Here's how the part is built. I have some questions about the finished solid (model axes, mm). Face numbers are marked on the shaded views. A direction names the side the tool comes from. Round coordinates to 2 decimals unless told otherwise and drop trailing zeros. Loops run counter-clockwise (first coordinate to the right, second up) from the corner with the lowest first, then second, coordinate; pieces in that order, holes last. Notation, with made-up numbers: M 67,10 L 126,10 A26 cw 126,41 Z; hole C -22,-33.75 d10. An arc over 180 degrees is marked long. Answer as a JSON object with one key per item and string values.
from build123d import *

# Parameters (mm, degrees)
SKETCH1_R           = 3.25
BOSS_EXTRUDE1_DEPTH = 2.25
SKETCH2_R           = 3.25
BOSS_EXTRUDE2_DEPTH = 5
SKETCH3_R           = 3.25
CUT_EXTRUDE1_DEPTH  = 26.744736797
FILLET1_R           = 5
CHAMFER1_SIZE       = 1
CUT_EXTRUDE2_REACH  = 52.824
SKETCH4_R           = 1.35
CHAMFER2_SIZE       = 0.75
CHAMFER2_SIZE2      = 2.060608065
CHAMFER3_SIZE       = 1


with BuildPart() as part:
    # Sketch1 → Boss-Extrude1 (new body, symmetric)
    with BuildSketch(Plane(origin=(0, 0, 0), x_dir=(0, 0, -1), z_dir=(1, 0, 0))):
        with BuildLine():
            Line((-1.775856455, 11.411388509), (3.7711595, 19.333348288))
            ThreePointArc((3.7711595, 19.333348288), (14.912987345, 21.297953152), (16.877592209, 10.156125306))
            Line((16.877592209, 10.156125306), (6.553216354, -4.588611491))
            ThreePointArc((6.553216354, -4.588611491), (3.693988906, -7.096086665), (0, -8))
            Line((0, -8), (-12.5, -8))
            Line((-12.5, -8), (-12.5, -3))
            Line((-12.5, -3), (-32.5, -3))
            Line((-32.5, -3), (-32.5, 8))
            Line((-32.5, 8), (-25, 8))
            Line((-25, 8), (-8.329072809, 8))
            ThreePointArc((-8.329072809, 8), (-4.635083903, 8.903913335), (-1.775856455, 11.411388509))
        make_face()
        Circle(SKETCH1_R, mode=Mode.SUBTRACT)
        with Locations((10.324375854, 14.744736797)):
            Circle(SKETCH1_R, mode=Mode.SUBTRACT)
    extrude(amount=BOSS_EXTRUDE1_DEPTH, both=True)

    # Sketch2 → Boss-Extrude2 (add)
    with BuildSketch(Plane(origin=(2.25, 0, 0), x_dir=(0, 0, -1), z_dir=(1, 0, 0))):
        with BuildLine():
            Line((-32.5, 8), (0, 8))
            ThreePointArc((0, 8), (8, 0), (0, -8))
            Line((0, -8), (-12.5, -8))
            Line((-12.5, -8), (-12.5, -3))
            Line((-12.5, -3), (-32.5, -3))
            Line((-32.5, -3), (-32.5, 8))
        make_face()
        Circle(SKETCH2_R, mode=Mode.SUBTRACT)
    boss_extrude2 = extrude(amount=BOSS_EXTRUDE2_DEPTH)

    # Mirror1: Boss-Extrude2 across plane
    add(boss_extrude2.mirror(Plane(origin=(0, 0, 0), x_dir=(0, 0, 1), z_dir=(1, 0, 0))))

    # Sketch3 → Cut-Extrude1 (cut, through all)
    with BuildSketch(Plane.XZ.offset(3)):
        with Locations((0, 25)):
            Circle(SKETCH3_R)
    extrude(amount=-CUT_EXTRUDE1_DEPTH, mode=Mode.SUBTRACT)

    # Fillet1
    fillet1_edges = [part.edges().sort_by_distance(p)[0] for p in [
        (7.25, 2.5, 32.5),
        (-7.25, 2.5, 32.5),
    ]]
    fillet(fillet1_edges, radius=FILLET1_R)

    # Chamfer1
    chamfer1_edges = [part.edges().sort_by_distance(p)[0] for p in [
        (0, 8, 32.5),
        (5.785533906, 8, 31.035533906),
        (-5.785533906, 8, 31.035533906),
        (-2.25, 14.744736797, -7.074375854),
        (2.25, 14.744736797, -7.074375854),
        (7.25, -8, 6.25),
        (7.25, 0, -8),
        (7.25, 8, 13.75),
        (7.25, 0, 3.25),
        (-7.25, 8, 13.75),
        (-7.25, 0, -8),
        (-7.25, -8, 6.25),
        (-7.25, 0, 3.25),
    ]]
    chamfer(chamfer1_edges, length=CHAMFER1_SIZE)

    # Sketch4 → Cut-Extrude2 (cut, up to next)
    with BuildSketch(Plane.XY.offset(32.5), mode=Mode.PRIVATE) as cut_extrude2_sk1:
        with Locations((0, 2)):
            Circle(SKETCH4_R)
    cut_extrude2_tool1 = extrude(cut_extrude2_sk1.sketch, amount=-CUT_EXTRUDE2_REACH, mode=Mode.PRIVATE) & part.part
    add(cut_extrude2_tool1.solids().sort_by_distance((0, 2, 32.5))[0], mode=Mode.SUBTRACT)

    # Chamfer2
    chamfer2_edges = [part.edges().sort_by_distance(p)[0] for p in [
        (-1.35, 2, 32.5),
    ]]
    chamfer2_side = [part.faces().sort_by_distance(p)[0] for p in [
        (-2.140341439, 2, 32.5),
    ]]
    chamfer(chamfer2_edges, length=CHAMFER2_SIZE, length2=CHAMFER2_SIZE2, reference=chamfer2_side[0])

    # Chamfer3
    chamfer3_edges = [part.edges().sort_by_distance(p)[0] for p in [
        (-3.25, -3, 25),
    ]]
    chamfer(chamfer3_edges, length=CHAMFER3_SIZE)


solid = part.part
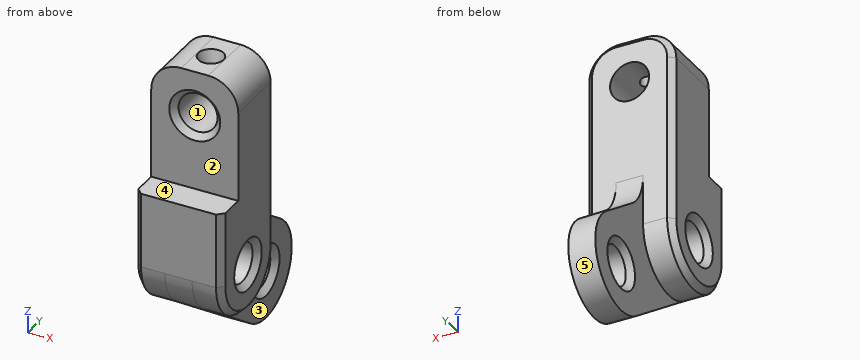
Item 1: If we mould it in two halves opening along X, with no side actions, what happens to the marked faces 1, 2 and 3? For each: pulls with the +X half, pulls with the -X half, needs draft (parallel to the pull), parting line crosses it, or undercut.
Resolved:
{"face 1": "undercut", "face 2": "needs draft", "face 3": "pulls with the +X half"}
Item 2: I want a section at B-B, the plane z = 25. Please give me the cut outline in (x, y), then the cut area to 3 significant figures.
Resolved:
{"outline": "M -7.25,-3 L -4.25,-3 L -3.25,-2 L -3.25,8 L -6.25,8 L -7.25,7 Z; M 3.25,-2 L 4.25,-3 L 7.25,-3 L 7.25,7 L 6.25,8 L 3.25,8 Z", "area": "86.0 mm²"}
Item 3: I'm going to push flat-ended pins straight in: pin 1 Ø6 at (x, z) = (-5.5, 24.5) entering from +Y; pin 2 Ø5.5 at (x, y) = (1, -6.5) entering from +Z; pin 3 Ø1 at (x, z) = (-2, 0) entering from +Y. Where does each tip first touch, or does it pass through?
Resolved:
{"pin 1": "y = 8", "pin 2": "z = 12.5", "pin 3": "y = 14.66"}
Item 4: I want a section at A-A, the plane x = 0. Please give me the cut outline in (y, z), then the cut area to 3 significant figures.
Resolved:
{"outline": "M -8,0 A8 ccw -4.59,-6.55 L 10.16,-16.88 A8 ccw 19.33,-3.77 L 11.41,1.78 A8 cw 8,8.33 L 8,21.75 L -2,21.75 L -3,20.75 L -3,12.5 L -8,12.5 Z; M -3,29.25 L -2,28.25 L 0.65,28.25 L 0.65,30.44 L -0.1,32.5 L -3,32.5 Z; M 3.35,28.25 L 8,28.25 L 8,31.5 L 7,32.5 L 4.1,32.5 L 3.35,30.44 Z; hole C 0,0 d6.5; hole C 14.74,-10.32 d6.5", "area": "656 mm²"}
Item 5: Please list where these lines run through material, in increasing order: probe 1 along Z at (x, y) = (1.5, 3); probe 2 along Y at (x, z) = (0, 29.6); probe 3 along Y at (x, z) = (3.5, 29.5). Write a range as from..to.
Resolved:
{"probe 1": "-11.87..-1.25, 1.25..22.12, 27.88..31.68", "probe 2": "-3..0.65, 3.35..8", "probe 3": "-3..8"}
Item 6: I want a section at C-C, the plane x = 2.75. State how many separate pieces and enclosed holes the cut face has, then the cut area to 3 significant figures.
Resolved:
{"separate pieces": "2", "enclosed holes": "1", "area": "447 mm²"}
Item 7: On a 3-axis mill with a long thin cutter (end or side, diameter ignored), from which of +Z, -Z, +X, -X, +Y, -Y can I reach the whole of each face in a straight line? I mean the marked faces 4 and 5. Say none if no direction works.
Resolved:
{"face 4": "+Z, +X, -X, -Y", "face 5": "+X, -X"}
